Build history of the part. All positions in model axes, mm. Give positions to 0.01 mm unless a question says otherwise; leave off trailing zeros. Write each loop counter-clockwise with the first axis right and the second up, starting at its lowest first coordinate (ties: lowest second). Pieces come first, ordered by that corner, then holes. Notation, with made-up numbers: (6, -23.5) -> (59, -23.5) arc R24 cw to (59, 8.5) -> close; hole circle Ø8 at (-18.75, 0.25). An arc over 180 degrees is marked (long way). One line per question, with ' | ' between items. Start each with the question number.
(1) Band-saw the part on C-C, the plane y = 3.1. Give the cut face in (x, z), and give its area (3 significant figures).
(2) Band-saw the part on A-A, the plane x = 61. Give the cut face in (y, z), and give its area (3 significant figures).
(3) Band-saw the part on B-B, the plane z = -29. Give the cut face in (x, y), and give its area (3 significant figures).
(4) Pin check, flat tips, straight feed: P1, Ø1.2, axis at y = 1.5, z = -43.5, coming from the +X side; P2, Ø2, axis at x = 2.5, y = 3, coming from the -Z side; P3, Ø2, axis at y = 2.5, z = -18.5, coming from the -X side. Stop position of each tip, or through.
(5) Drill centre lines: probe 1 along X at (y, z) = (0.8, -29); probe 2 along X at (y, z) = (2.6, -20.25); probe 3 along Z at (x, y) = (57.5, 1.65). Where is each one in solid material? Low to high. Write a range as from..to.
(6) Band-saw the part on D-D, the plane x = 41. Give the cut face in (y, z), and give its area (3 significant figures).
from build123d import *

# Parameters (mm, degrees)
SKETCH1_W           = 80
SKETCH1_H           = 75
BOSS_EXTRUDE1_DEPTH = 4
SKETCH2_R           = 6
SKETCH2_R_2         = 1.5
CUT_EXTRUDE1_DEPTH  = 110.731490467
SKETCH3_W           = 26
SKETCH3_H           = 6
SKETCH3_W_2         = 4
SKETCH3_H_2         = 25
CUT_EXTRUDE2_DEPTH  = 110.731490467


with BuildPart() as part:
    # Sketch1 → Boss-Extrude1 (new body)
    with BuildSketch(Plane(origin=(0, 0, 0), x_dir=(1, 0, 0), z_dir=(0, 1, 0))):
        with Locations((40, 37.5)):
            Rectangle(SKETCH1_W, SKETCH1_H)
    extrude(amount=BOSS_EXTRUDE1_DEPTH)

    # Sketch2 → Cut-Extrude1 (cut, through all)
    with BuildSketch(Plane(origin=(0, 4, 0), x_dir=(1, 0, 0), z_dir=(0, 1, 0))):
        with Locations(Location((41, 29, 0), (0, 0, 270))):
            Circle(SKETCH2_R)
        with Locations(Location((61, 37.75, 0), (0, 0, 270))):
            Circle(SKETCH2_R_2)
        with Locations(Location((61, 20.25, 0), (0, 0, 270))):
            Circle(SKETCH2_R_2)
    extrude(amount=-CUT_EXTRUDE1_DEPTH, mode=Mode.SUBTRACT)

    # Sketch3 → Cut-Extrude2 (cut, through all)
    with BuildSketch(Plane(origin=(0, 4, 0), x_dir=(1, 0, 0), z_dir=(0, 1, 0))):
        with Locations((67, 3)):
            Rectangle(SKETCH3_W, SKETCH3_H)
        with Locations((78, 37.5)):
            Rectangle(SKETCH3_W_2, SKETCH3_H_2)
        with Locations((67, 72)):
            Rectangle(SKETCH3_W, SKETCH3_H)
        Polygon((0, 75), (0, 50), (6, 50), (6, 69), (26, 69), (26, 75), align=None)
        Polygon((6, 25), (0, 25), (0, 0), (26, 0), (26, 6), (6, 6), align=None)
    extrude(amount=-CUT_EXTRUDE2_DEPTH, mode=Mode.SUBTRACT)


solid = part.part
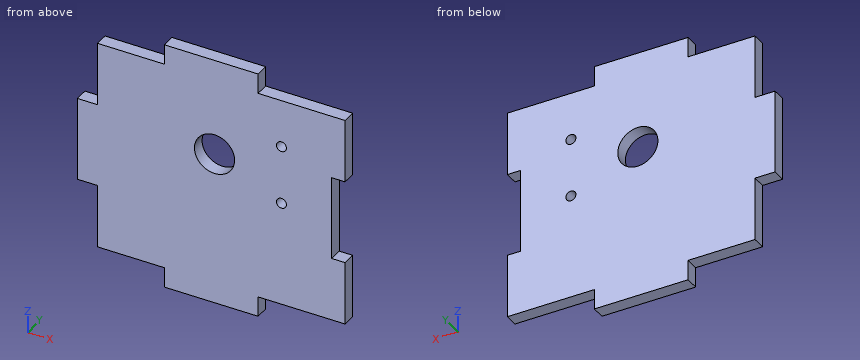
Results:
1) outline: (0, -50) -> (6, -50) -> (6, -69) -> (26, -69) -> (26, -75) -> (54, -75) -> (54, -69) -> (80, -69) -> (80, -50) -> (76, -50) -> (76, -25) -> (80, -25) -> (80, -6) -> (54, -6) -> (54, 0) -> (26, 0) -> (26, -6) -> (6, -6) -> (6, -25) -> (0, -25) -> close; hole circle Ø12 at (41, -29); hole circle Ø3 at (61, -37.75); hole circle Ø3 at (61, -20.25) | area: 4,920 mm²
2) outline: (0, -69) -> (4, -69) -> (4, -39.25) -> (0, -39.25) -> close; (0, -36.25) -> (4, -36.25) -> (4, -21.75) -> (0, -21.75) -> close; (0, -18.75) -> (4, -18.75) -> (4, -6) -> (0, -6) -> close | area: 228 mm²
3) outline: (0, 0) -> (35, 0) -> (35, 4) -> (0, 4) -> close; (47, 0) -> (76, 0) -> (76, 4) -> (47, 4) -> close | area: 256 mm²
4) P1: stops at x = 76 | P2: stops at z = -50 | P3: stops at x = 6
5) probe 1: x = 0..35, 47..76 | probe 2: x = 6..59.5, 62.5..80 | probe 3: z = -69..-6
6) outline: (0, -75) -> (4, -75) -> (4, -35) -> (0, -35) -> close; (0, -23) -> (4, -23) -> (4, 0) -> (0, 0) -> close | area: 252 mm²
